Here's the drawing with two shaded views (mm, measured from the low corner). I have some questions. A direction names the side the tool comes from. Round coordinates to 2 decimals unless told otherwise and drop trailing zeros. Loops run counter-clockwise (first coordinate to the right, second up) from the corner with the lowest first, then second, coordinate; pieces in that order, holes last.
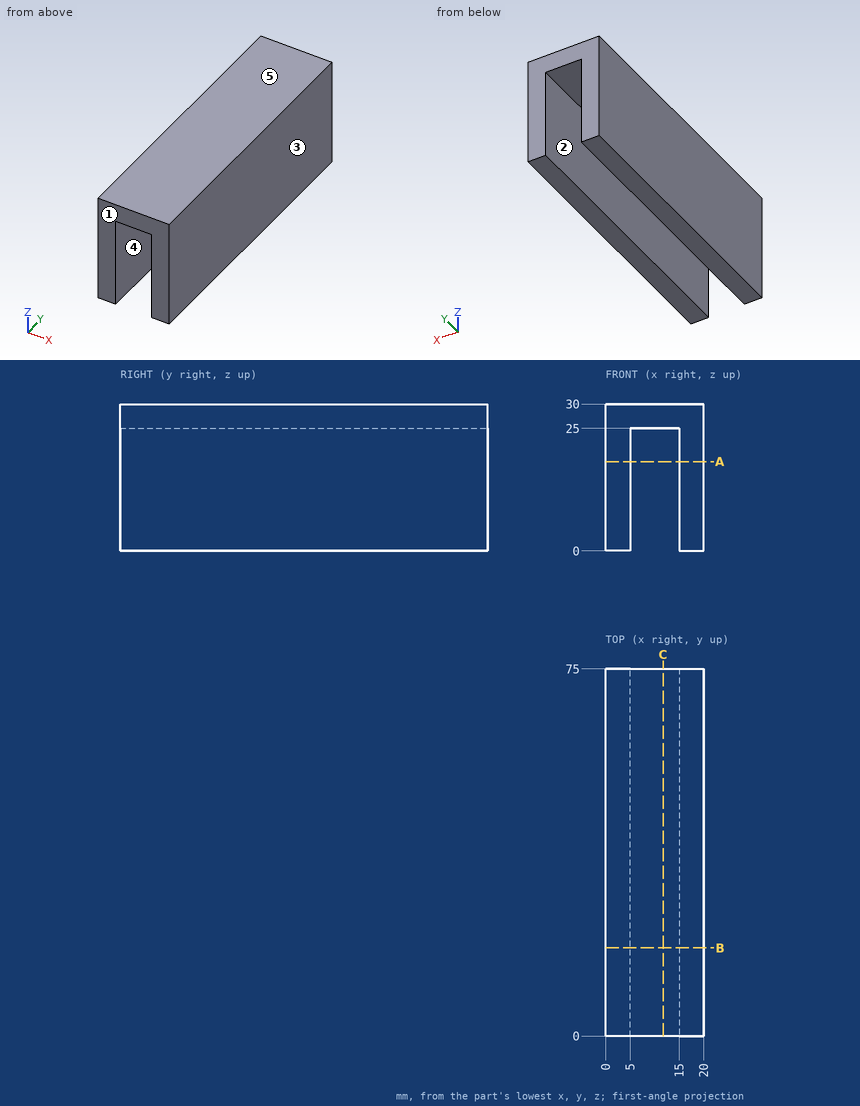
Item 1: For the marked faces 1 and 2, which set-ups out of +Z, -Z, +X, -X, +Y, -Y let a thin tool reach every point of the face, with its end or its side?
Results list:
face 1: +Z, -Z, +X, -X, -Y
face 2: -Z, +Y, -Y
Item 2: Will this pin go through, and if not, where does the flat tip stop? pin 1 (2 mm diameter, centred on x = 12.5, y = 66.5, fed in from -Z).
Results list:
pin 1: stops at z = 25
Item 3: If we section it at A-A, the plane z = 18.25: Please give me the cut outline in (x, y).
Results list:
outline: (0, 0) - (5, 0) - (5, 75) - (0, 75) - close; (15, 0) - (20, 0) - (20, 75) - (15, 75) - close
Item 4: If we section it at B-B, the plane y = 18: Please give me the cut outline in (x, z), then the cut area to 3 significant figures.
Results list:
outline: (0, 0) - (5, 0) - (5, 25) - (15, 25) - (15, 0) - (20, 0) - (20, 30) - (0, 30) - close
area: 350 mm2
Item 5: We'd pull the mould along X, two halves only. Please class the marked faces 3, 4 and 5: released by +X, released by -X, zero draft, split by the parting line, or undercut.
Results list:
face 3: released by +X
face 4: undercut
face 5: zero draft
Item 6: If I drill on line 1 along X through (y, z) = (39.5, 15); line 2 along Z through (x, y) = (5.5, 16), over which ranges is the centre line in solid material (lowest first)?
Results list:
line 1: x = 0 to 5, 15 to 20
line 2: z = 25 to 30
Item 7: If we section it at C-C, the plane x = 11.75: Please give me the cut outline in (y, z).
Results list:
outline: (0, 25) - (75, 25) - (75, 30) - (0, 30) - close
